Print and shaded views of the part. All mm, measured from the part's lowest x, y and z. Round coordinates to 2 decimals unless told otherwise and drop trailing zeros. Write each loop counter-clockwise with the first axis right and the second up, starting at its lowest first coordinate (ties: lowest second). Pieces come first, ordered by that corner, then holes.
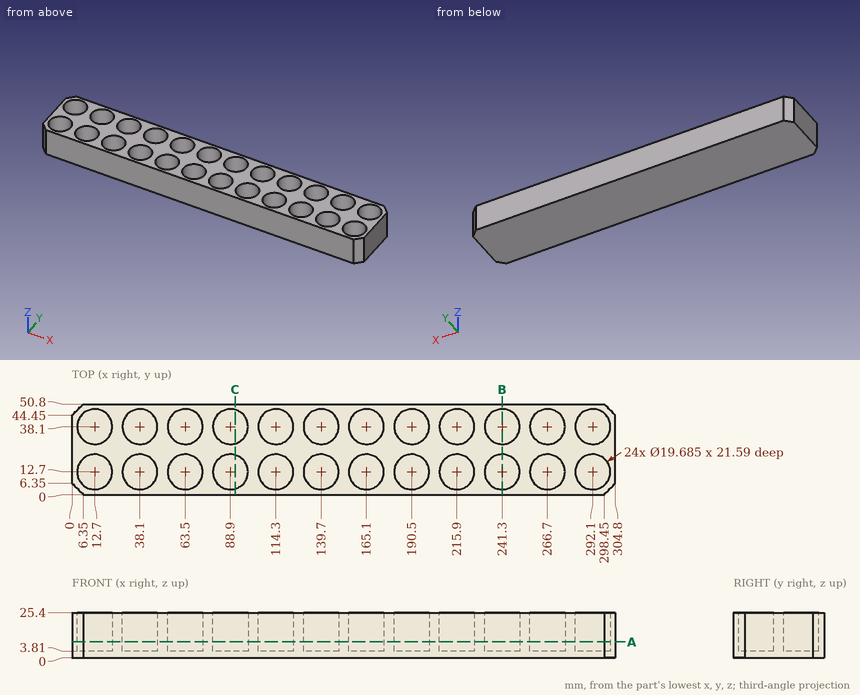
1) Wall check: L1, parallel to Y at x = 191.5, z = 16.25; L2, parallel to Y at x = 156, z = 24; L3, parallel to Z at x = 249.5, y = 39.5. Give the ranges that are in metal, low to high.
Results:
L1: y = 0 to 2.91, 22.49 to 28.31, 47.89 to 50.8
L2: y = 0 to 8.95, 16.45 to 34.35, 41.85 to 50.8
L3: z = 0 to 3.81
2) Slice it at C-C (x = 91.5). Write the cut outline in (y, z), plus the area to 3 significant figures.
Results:
outline: (0, 0) - (50.8, 0) - (50.8, 25.4) - (47.59, 25.4) - (47.59, 3.81) - (28.61, 3.81) - (28.61, 25.4) - (22.19, 25.4) - (22.19, 3.81) - (3.21, 3.81) - (3.21, 25.4) - (0, 25.4) - close
area: 471 mm2
3) Slice it at B-B (x = 241.3). Write the cut outline in (y, z), plus the area to 3 significant figures.
Results:
outline: (0, 0) - (50.8, 0) - (50.8, 25.4) - (47.94, 25.4) - (47.94, 3.81) - (28.26, 3.81) - (28.26, 25.4) - (22.54, 25.4) - (22.54, 3.81) - (2.86, 3.81) - (2.86, 25.4) - (0, 25.4) - close
area: 440 mm2
4) Pin check, flat tip, straight feed: pin 1 Ø6 at (x, y) = (33.5, 43) entering from +Z. Stop position of the tip, or through.
Results:
pin 1: stops at z = 3.81
5) Slice it at A-A (z = 9). Count the separate pieces of the cut face and the enclosed holes in it, plus the area to 3 significant figures.
Results:
separate pieces: 1
enclosed holes: 24
area: 8,100 mm2
